Autodesk Inventor part; units mm, degrees
ref_plane "YZ Plane" through (0, 0, 0) normal (1, 0, 0) x (0, 1, 0)
ref_plane "XZ Plane" through (0, 0, 0) normal (0, 1, 0) x (-1, 0, 0)
ref_plane "XY Plane" through (0, 0, 0) normal (0, 0, 1) x (1, 0, 0)
sketch "Sketch1" plane through (0, 0, 0) normal (0, 1, 0) x (-1, 0, 0)
  line L0 (0, 0) -> (220, 0)
  line L1 (220, 0) -> (220, 70)
  line L2 (220, 70) -> (0, 70)
  line L3 (0, 70) -> (0, 0)
  line L4 (16, 51) -> (114, 51) construction
  line L5 (114, 51) -> (114, 11) construction
  line L6 (114, 11) -> (16, 11) construction
  line L7 (16, 11) -> (16, 51) construction
  line L8 (15.5, 51.5) -> (114.5, 51.5)
  line L9 (114.5, 51.5) -> (114.5, 10.5)
  line L10 (114.5, 10.5) -> (15.5, 10.5)
  line L11 (15.5, 10.5) -> (15.5, 51.5)
  circle A0 centre (139, 55) radius 1.5
  circle A1 centre (139, 37.5) radius 5.5
  circle A2 centre (139, 22) radius 3
  line L12 (2, 65) -> (152, 65) construction
  line L13 (152, 65) -> (152, 10) construction
  line L14 (152, 10) -> (2, 10) construction
  line L15 (2, 10) -> (2, 65) construction
  point P0 (65, 51.5)
  point P1 (65, 51)
  point P2 (114, 31)
  point P3 (114.5, 31)
  dimension "d11" = 220
  dimension "d106" = 40
  dimension "d107" = 98
  dimension "d108" = 99
  dimension "d109" = 41
  dimension "d110" = 25
  dimension "d111" = 6
  dimension "d112" = 15.5
  dimension "d113" = 17.5
  dimension "d114" = 13.5
  dimension "d115" = 3
  dimension "d116" = 11
  dimension "d117" = 55
  dimension "d118" = 150
  dimension "d119" = 14
  dimension "d120" = 14
  dimension "d121" = 5
  dimension "d122" = 2
  dimension "d123" = 10
extrude "Extrusion8" add sketch "Sketch1" along normal blind 6
sketch "Sketch7" plane through (0, 6, 0) normal (0, 1, 0) x (1, 0, 0)
  line L0 (0, 0) -> (-220, 0)
  line L1 (-220, 0) -> (-220, -70)
  line L2 (-220, -70) -> (0, -70)
  line L3 (0, -70) -> (0, 0)
  line L4 (-220, -15) -> (-224, -15)
  line L5 (-226, -17) -> (-226, -21)
  line L6 (-224, -23) -> (-220, -23)
  line L7 (-220, -23) -> (-220, -15)
  line L8 (-220, -47) -> (-224, -47)
  line L9 (-226, -49) -> (-226, -53)
  line L10 (-224, -55) -> (-220, -55)
  line L11 (-220, -55) -> (-220, -47)
  line L12 (0, -15) -> (4, -15)
  line L13 (6, -17) -> (6, -21)
  line L14 (4, -23) -> (0, -23)
  line L15 (0, -23) -> (0, -15)
  line L16 (0, -47) -> (4, -47)
  line L17 (6, -49) -> (6, -53)
  line L18 (4, -55) -> (0, -55)
  line L19 (0, -55) -> (0, -47)
  arc A0 (-224, -15) -> (-226, -17) centre (-224, -17) ccw
  arc A1 (-226, -21) -> (-224, -23) centre (-224, -21) ccw
  arc A2 (-224, -47) -> (-226, -49) centre (-224, -49) ccw
  arc A3 (-226, -53) -> (-224, -55) centre (-224, -53) ccw
  arc A4 (6, -17) -> (4, -15) centre (4, -17) ccw
  arc A5 (4, -23) -> (6, -21) centre (4, -21) ccw
  arc A6 (6, -49) -> (4, -47) centre (4, -49) ccw
  arc A7 (4, -55) -> (6, -53) centre (4, -53) ccw
  dimension "d126" = 2
  dimension "d127" = 15
  dimension "d128" = 8
  dimension "d129" = 8
  dimension "d130" = 15
  dimension "d131" = 6
  dimension "d132" = 6
extrude "Extrusion9" add sketch "Sketch7" against normal blind 6 contours L12 A4 L13 A5 L14 L3 | L1 L6 A1 L5 A0 L4 | L16 A6 L17 A7 L18 L3 | L1 L10 A3 L9 A2 L8
properties part number "front_panel_2004_display"
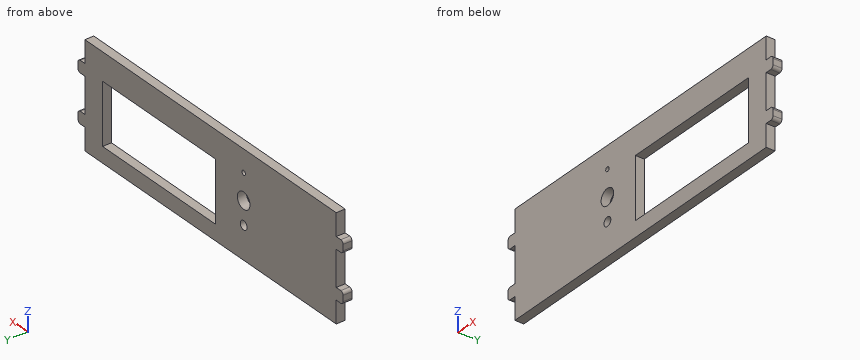
Geometry check sheet. Reference: the model listing, model coordinates, mm. Give positions to 0.01 mm unless a question says otherwise; leave off trailing zeros. Order: outer loops, then holes, each group sorted by start corner. A loop starts at its lowest first (then second) coordinate and runs counter-clockwise, first axis right, second up. Notation, with made-up numbers: (24.25, 74.5) - (63.25, 74.5) arc R27 cw to (63.25, 91.5) - close; hole circle Ø7 at (24.5, -28). An arc over 180 degrees is marked (long way). Write item = value, one per line. Start each with the question number.
1) Section check D-D (z = 63). Enter the section's corners in (x, y).
2) Scan lines: L1, parallel to Z at x = -139, y = 2.4; L2, parallel to X at y = 2.2, z = 37; L3, parallel to Z at x = -96.5, y = 5.7. Record each from-to range of solid material in increasing order.
3) Section check A-A (x = -73.5). Enter the section's corners in (y, z).
4) Section check B-B (z = 37.5). Enter the section's corners in (x, y), then the cut area to 3 significant figures.
5) Section check C-C (y = 1.5). Count the separate pieces of the cut face and the enclosed holes in it, then the cut area to 3 significant figures.
6) Gauge pin test, flat ends, axial feed: pin 1 Ø6 at (x, z) = (-167.5, 39) entering from -Y; pin 2 Ø1.8 at (y, z) = (2.5, 6.5) entering from -X; pin 3 Ø2 at (x, y) = (3, 3.5) entering from -Z; pin 4 Ø5.5 at (x, z) = (-139, 22) entering from +Y. Record the tip position at first contact, or that the pin passes through.
Geometry check:
q1.outline = (-220, 0) - (0, 0) - (0, 6) - (-220, 6) - close
q2.L1 = 0 to 19, 25 to 32, 43 to 53.5, 56.5 to 70
q2.L2 = -220 to -144.48, -133.52 to -114.5, -15.5 to 0
q2.L3 = 0 to 10.5, 51.5 to 70
q3.outline = (0, 0) - (6, 0) - (6, 10.5) - (0, 10.5) - close; (0, 51.5) - (6, 51.5) - (6, 70) - (0, 70) - close
q4.outline = (-220, 0) - (-144.5, 0) - (-144.5, 6) - (-220, 6) - close; (-133.5, 0) - (-114.5, 0) - (-114.5, 6) - (-133.5, 6) - close; (-15.5, 0) - (0, 0) - (0, 6) - (-15.5, 6) - close
q4.area = 660 mm2
q5.separate_pieces = 1
q5.enclosed_holes = 4
q5.area = 11,400 mm2
q6.pin_1 = 0
q6.pin_2 = -220
q6.pin_3 = 15
q6.pin_4 = through
